Check sheet for the modelled part. Datum: model origin and axes. Units: mm. Give positions to 0.01 mm unless a question says otherwise; leave off trailing zeros. Loops run counter-clockwise (first coordinate to the right, second up) from the corner with the lowest first, then second, coordinate; pieces in that order, holes last. Notation, with made-up numbers: (-17.5, -30) -> (16.5, -30) arc R18 cw to (16.5, 5) -> close; hole circle Ø4 at (77, 68.5). An arc over 180 degrees is marked (long way). Write each question's results on one line, items separated by ' | '. Start each with the question number.
1. Cross-section at D-D on x = 197. Record the boundary of the cut face in (y, z).
2. Gauge pin test, flat ends, axial feed: pin 1 Ø5 at (x, y) = (235, 0) entering from +Z; pin 2 Ø4 at (x, z) = (66, 11) entering from +Y; pin 3 Ø8 at (x, z) = (115.5, 14) entering from +Y; pin 4 Ø5 at (y, z) = (99.5, 15) entering from +X. Record the tip position at first contact, or that the pin passes through.
3. Cross-section at B-B on z = 14.25. Record the boundary of the cut face in (x, y), and give its area (3 significant figures).
4. Cross-section at A-A on x = 0. Record the boundary of the cut face in (y, z), and give its area (3 significant figures).
5. Cross-section at C-C on y = -75. Record the boundary of the cut face in (x, z), and give its area (3 significant figures).
6. Mould release check, pull along X, two halves, no side actions. Record for faces 1 (the face through (54, 4, 0)), 2 (the face through (6.466, -2.681, 8.874)), 3 (the face through (247.994, 78.097, 8.874)): +X half, -X half, draft (parallel to the pull), parting line (faces both ways), or undercut.
7. Material ranges on L1, parallel to Y at x = 0, z = 14; L2, parallel to Y at x = -117.5, z = 8.5; L3, parallel to Y at x = -90.5, z = 13.5, recorded low to high. Write a range as from..to.
from build123d import *

# Parameters (mm, degrees)
SKETCH_R           = 260
PAD_DEPTH          = 18
SKETCH001_R        = 2
POCKET_DEPTH       = 1489.223621
POLARPATTERN_COUNT = 3
SKETCH002_R        = 7
POCKET001_DEPTH    = 18.001


with BuildPart() as part:
    # Sketch → Pad (new body)
    with BuildSketch(Plane.XY):
        Circle(SKETCH_R)
    extrude(amount=PAD_DEPTH)

    # Sketch001 (on Face3 of Pad) → Pocket (cut, through all)
    with BuildSketch(Plane.XY.offset(18)):
        with Locations((235, 0)):
            Circle(SKETCH001_R)
    pocket = extrude(amount=-POCKET_DEPTH, mode=Mode.SUBTRACT)

    # PolarPattern: Pocket ×3 about axis
    polarpattern_axis = Axis((0, 0, 18), (0, 0, 1))
    for i in range(1, POLARPATTERN_COUNT):
        add(pocket.rotate(polarpattern_axis, i * 360 / POLARPATTERN_COUNT), mode=Mode.SUBTRACT)

    # Sketch002 → Pocket001 (cut, through all)
    with BuildSketch(Plane.XY):
        Circle(SKETCH002_R)
    extrude(amount=POCKET001_DEPTH, mode=Mode.SUBTRACT)


solid = part.part
Geometry says:
1) outline: (-169.68, 0) -> (169.68, 0) -> (169.68, 18) -> (-169.68, 18) -> close
2) pin 1: z = 18 | pin 2: y = 252 | pin 3: y = 234.88 | pin 4: x = 241.23
3) outline: circle Ø520 at (0, 0); hole circle Ø4 at (-117.5, -203.52); hole circle Ø4 at (-117.5, 203.52); hole circle Ø14 at (0, 0); hole circle Ø4 at (235, 0) | area: 212,000 mm^2
4) outline: (-260, 0) -> (-7, 0) -> (-7, 18) -> (-260, 18) -> close; (7, 0) -> (260, 0) -> (260, 18) -> (7, 18) -> close | area: 9,110 mm^2
5) outline: (-248.95, 0) -> (248.95, 0) -> (248.95, 18) -> (-248.95, 18) -> close | area: 8,960 mm^2
6) face 1: draft | face 2: undercut | face 3: parting line
7) L1: -260..-7, 7..260 | L2: -231.93..-205.52, -201.52..201.52, 205.52..231.93 | L3: -243.74..243.74
